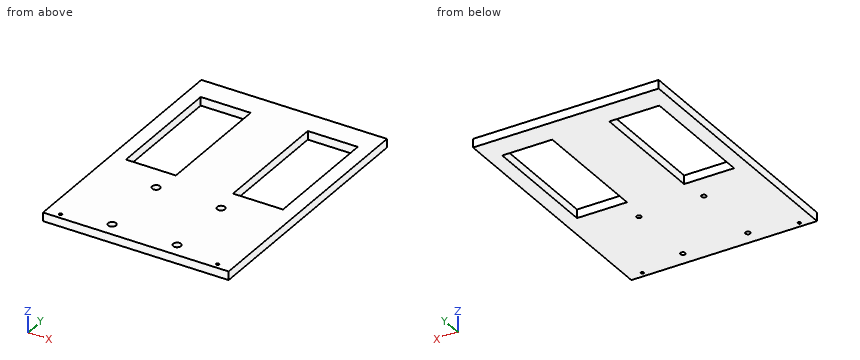
```python
from build123d import *

# Parameters (mm, degrees)
SKETCH1_W               = 260
SKETCH1_H               = 360
BOSS_EXTRUDE1_DEPTH     = 12
CUT_EXTRUDE1_DEPTH      = 550.727205075
CUT_EXTRUDE1_DEPTH_BACK = 550.727205075
SKETCH2_R               = 3.3
SKETCH3_R               = 5.5
CUT_EXTRUDE3_DEPTH      = 6.5
CUT_EXTRUDE4_DEPTH      = 550.727205075
CUT_EXTRUDE4_DEPTH_BACK = 550.727205075
SKETCH4_R               = 2.1
CUT_EXTRUDE5_DEPTH      = 550.727205075
CUT_EXTRUDE5_DEPTH_BACK = 550.727205075
SKETCH5_W               = 70
SKETCH5_H               = 170


with BuildPart() as part:
    # Sketch1 → Boss-Extrude1 (new body)
    with BuildSketch(Plane.XY):
        with Locations((0, 354)):
            Rectangle(SKETCH1_W, SKETCH1_H)
    extrude(amount=BOSS_EXTRUDE1_DEPTH)

    # Sketch2 → Cut-Extrude1 (cut, two sides: drawn at the far end of the back side and taken through both)
    with BuildSketch(Plane.XY.offset(-CUT_EXTRUDE1_DEPTH_BACK)):
        with Locations((-45.5, 194)):
            Circle(SKETCH2_R)
        with Locations((-45.5, 294)):
            Circle(SKETCH2_R)
        with Locations((45.5, 194)):
            Circle(SKETCH2_R)
        with Locations((45.5, 294)):
            Circle(SKETCH2_R)
    extrude(amount=CUT_EXTRUDE1_DEPTH + CUT_EXTRUDE1_DEPTH_BACK, mode=Mode.SUBTRACT)

    # Sketch3 → Cut-Extrude3 (cut)
    with BuildSketch(Plane.XY.offset(12)):
        with Locations((-45.5, 194)):
            Circle(SKETCH3_R)
        with Locations((-45.5, 294)):
            Circle(SKETCH3_R)
        with Locations((45.5, 194)):
            Circle(SKETCH3_R)
        with Locations((45.5, 294)):
            Circle(SKETCH3_R)
    extrude(amount=-CUT_EXTRUDE3_DEPTH, mode=Mode.SUBTRACT)

    # Sketch4 → Cut-Extrude4 (cut, two sides: drawn at the far end of the back side and taken through both)
    with BuildSketch(Plane.XY.offset(-CUT_EXTRUDE4_DEPTH_BACK)):
        with Locations((-110, 181.5)):
            Circle(SKETCH4_R)
        with Locations((110, 181.5)):
            Circle(SKETCH4_R)
    extrude(amount=CUT_EXTRUDE4_DEPTH + CUT_EXTRUDE4_DEPTH_BACK, mode=Mode.SUBTRACT)

    # Sketch5 → Cut-Extrude5 (cut, two sides: drawn at the far end of the back side and taken through both)
    with BuildSketch(Plane.XY.offset(-CUT_EXTRUDE5_DEPTH_BACK)):
        with Locations((-75, 415)):
            Rectangle(SKETCH5_W, SKETCH5_H)
        with Locations((75, 415)):
            Rectangle(SKETCH5_W, SKETCH5_H)
    extrude(amount=CUT_EXTRUDE5_DEPTH + CUT_EXTRUDE5_DEPTH_BACK, mode=Mode.SUBTRACT)


solid = part.part
```
Could you check a few things on this model? Use its own coordinates, in mm. Round coordinates to 2 decimals unless told otherwise and drop trailing zeros. Loops run counter-clockwise (first coordinate to the right, second up) from the corner with the lowest first, then second, coordinate; pieces in that order, holes last.
Q1. I want a section at B-B (x = -82). Write out the boundary of the cut face in (y, z).
Q2. I want a section at A-A (y = 381). Write out the boundary of the cut face in (x, z).
Q3. Please list where these lines run through material, in increasing order: L1, parallel to Y at x = 45.5, z = 9.25; L2, parallel to Y at x = -45.5, z = 1.45; L3, parallel to X at y = 294, z = 3.75.
Q4. For P1, Ø3.5, axis at x = 47.5, y = 292, coming from the +Z side, with a flat end and sliding along its axis, tell me the tip position at first contact or that it passes through.
Answer below:
1. outline: (174, 0) - (330, 0) - (330, 12) - (174, 12) - close; (500, 0) - (534, 0) - (534, 12) - (500, 12) - close
2. outline: (-130, 0) - (-110, 0) - (-110, 12) - (-130, 12) - close; (-40, 0) - (40, 0) - (40, 12) - (-40, 12) - close; (110, 0) - (130, 0) - (130, 12) - (110, 12) - close
3. L1: y = 174 to 188.5, 199.5 to 288.5, 299.5 to 330, 500 to 534
3. L2: y = 174 to 190.7, 197.3 to 290.7, 297.3 to 330, 500 to 534
3. L3: x = -130 to -48.8, -42.2 to 42.2, 48.8 to 130
4. P1: stops at z = 5.5
